Verification items for the finished model (mm, model axes). Face numbers are marked on the shaded views. A direction names the side the tool comes from. Round coordinates to 2 decimals unless told otherwise and drop trailing zeros. Write each loop counter-clockwise with the first axis right and the second up, starting at its lowest first coordinate (ties: lowest second). Pieces come first, ordered by that corner, then holes. Notation, with made-up numbers: (76.25, 62) -> (111.25, 62) arc R15 ccw to (111.25, 86) -> close; hole circle Ø6 at (-1.5, 88). An arc over 180 degrees is marked (long way). Answer as a JSON object with one key per item and string values. Group by question number.
(1) Gauge pin test, flat ends, axial feed: pin 1 Ø6 at (x, y) = (13.5, 41) entering from -Z; pin 2 Ø1.6 at (x, z) = (34.5, -47.5) entering from +Y; pin 3 Ø12 at (y, z) = (38.5, -49.5) entering from -X; pin 4 Ø10 at (x, z) = (22, -36) entering from -Y. Record the tip position at first contact, or that the pin passes through.
(2) Sectioned sample at B-B on z = -33.5. Record the cut outline in (x, y), and give its area (3 significant figures).
(3) Sectioned sample at C-C on x = 14.5. Record the cut outline in (y, z), and give its area (3 significant figures).
(4) Scan lines: L1, parallel to X at y = 42.75, z = -55.5; L2, parallel to Y at x = 14.5, z = -49; L3, parallel to X at y = 48.75, z = -42. Record each from-to range of solid material in increasing order. Write a range as from..to.
(5) Sectioned sample at A-A on x = 7. Record the cut outline in (y, z).
(6) Draft check along X on the marked faces 4, 5 and 6. Enter one of: released by +X, released by -X, zero draft, split by the parting line, or undercut.
(7) Set-up check for the marked faces 1, 2 and 3: record each of +Z, -Z, +X, -X, +Y, -Y from which the full face is reachable in a straight line by a thin tool's end or side.
(8) Sectioned sample at D-D on y = 51. Record the cut outline in (x, z), and give its area (3 significant figures).
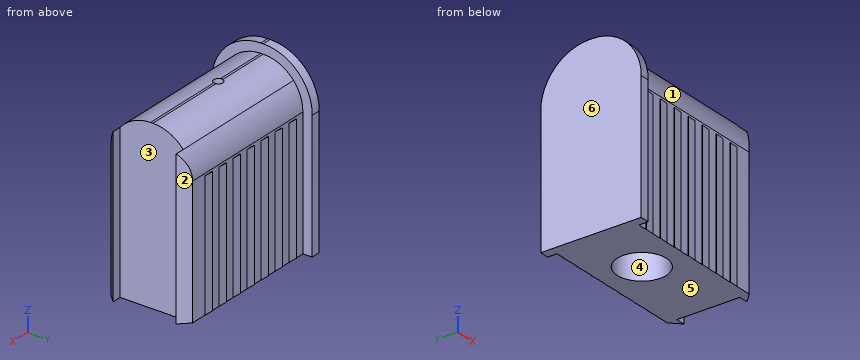
```python
from build123d import *

# Parameters (mm, degrees)
F1_DEPTH = 35.5
F2_DEPTH = 2
F3_DEPTH = 33.5
F4_R     = 5.25
F4_R_2   = 1
F5_DEPTH = 25
F6_DEPTH = 36
F7_DEPTH = 32.9782255751
F8_DEPTH = 27


with BuildPart() as f1:
    # F0 (on Right) → F1 (new body)
    with BuildSketch(Plane.YZ):
        with BuildLine():
            Line((49.4756655051, -63.7959514514), (51.4756655051, -63.7959514514))
            Line((51.4756655051, -63.7959514514), (51.4756655051, -36.2959514514))
            ThreePointArc((51.4756655051, -36.2959514514), (50.9600252165, -33.3804755039), (49.4756655051, -30.8187258763))
            Line((49.4756655051, -30.8187258763), (49.4756655051, -63.7959514514))
        make_face()
    extrude(amount=F1_DEPTH)



with BuildPart() as f1b:
    # F0 (on Right) → F1, piece 2 (new body)
    with BuildSketch(Plane.YZ):
        with BuildLine():
            Line((33.9756655051, -63.7959514514), (35.9756655051, -63.7959514514))
            Line((35.9756655051, -63.7959514514), (35.9756655051, -30.8187258763))
            ThreePointArc((35.9756655051, -30.8187258763), (34.4913057938, -33.3804755039), (33.9756655051, -36.2959514514))
            Line((33.9756655051, -36.2959514514), (33.9756655051, -63.7959514514))
        make_face()
    extrude(amount=F1_DEPTH)


with BuildPart() as f1_1:
    add(f1.part)

    add(f1b.part)  # F2 merges F1b
    # F0 (on Right) → F2 (join)
    with BuildSketch(Plane.YZ):
        with BuildLine():
            Line((51.4756655051, -36.2959514514), (51.4756655051, -63.7959514514))
            Line((51.4756655051, -63.7959514514), (53.4756655051, -63.7959514514))
            Line((53.4756655051, -63.7959514514), (53.4756655051, -36.2959514514))
            ThreePointArc((53.4756655051, -36.2959514514), (50.4002867076, -28.8713302489), (42.9756655051, -25.7959514514))
            Line((42.9756655051, -25.7959514514), (42.4756655051, -25.7959514514))
            ThreePointArc((42.4756655051, -25.7959514514), (35.0510443027, -28.8713302489), (31.9756655051, -36.2959514514))
            Line((31.9756655051, -36.2959514514), (31.9756655051, -63.7959514514))
            Line((31.9756655051, -63.7959514514), (33.9756655051, -63.7959514514))
            Line((33.9756655051, -63.7959514514), (33.9756655051, -36.2959514514))
            ThreePointArc((33.9756655051, -36.2959514514), (34.4913057938, -33.3804755039), (35.9756655051, -30.8187258763))
            ThreePointArc((35.9756655051, -30.8187258763), (38.8914234226, -28.5886037432), (42.4756655051, -27.7959514514))
            Line((42.4756655051, -27.7959514514), (42.9756655051, -27.7959514514))
            ThreePointArc((42.9756655051, -27.7959514514), (46.5599075877, -28.5886037432), (49.4756655051, -30.8187258763))
            ThreePointArc((49.4756655051, -30.8187258763), (50.9600252165, -33.3804755039), (51.4756655051, -36.2959514514))
        make_face()
        with BuildLine():
            Line((35.9756655051, -63.7959514514), (49.4756655051, -63.7959514514))
            Line((49.4756655051, -63.7959514514), (49.4756655051, -30.8187258763))
            ThreePointArc((49.4756655051, -30.8187258763), (46.5599075877, -28.5886037432), (42.9756655051, -27.7959514514))
            Line((42.9756655051, -27.7959514514), (42.4756655051, -27.7959514514))
            ThreePointArc((42.4756655051, -27.7959514514), (38.8914234226, -28.5886037432), (35.9756655051, -30.8187258763))
            Line((35.9756655051, -30.8187258763), (35.9756655051, -63.7959514514))
        make_face()
    extrude(amount=F2_DEPTH)

    # F0 (on Right) → F3 (join)
    with BuildSketch(Plane.YZ):
        with BuildLine():
            Line((35.9756655051, -63.7959514514), (49.4756655051, -63.7959514514))
            Line((49.4756655051, -63.7959514514), (49.4756655051, -30.8187258763))
            ThreePointArc((49.4756655051, -30.8187258763), (46.5599075877, -28.5886037432), (42.9756655051, -27.7959514514))
            Line((42.9756655051, -27.7959514514), (42.4756655051, -27.7959514514))
            ThreePointArc((42.4756655051, -27.7959514514), (38.8914234226, -28.5886037432), (35.9756655051, -30.8187258763))
            Line((35.9756655051, -30.8187258763), (35.9756655051, -63.7959514514))
        make_face()
    extrude(amount=F3_DEPTH)

    # F4 (on face) → F5 (cut)
    with BuildSketch(Plane(origin=(0, 0, -63.7959514514), x_dir=(1, 0, 0), z_dir=(0, 0, -1))):
        with Locations((14.5, -42.7256655051)):
            Circle(F4_R)
        with Locations((14.5, -42.7256655051)):
            Circle(F4_R_2, mode=Mode.SUBTRACT)
    extrude(amount=-F5_DEPTH, mode=Mode.SUBTRACT)

    # F6 (cut, through all): a face of the model
    f6_faces = [f1_1.faces().sort_by_distance(p)[0] for p in [
        (14.5, 42.7256655051, -63.7959514514),
    ]]
    extrude(f6_faces, amount=-F6_DEPTH, mode=Mode.SUBTRACT)

    # F4 (on face) → F7 (cut, through all)
    with BuildSketch(Plane(origin=(0, 0, -63.7959514514), x_dir=(1, 0, 0), z_dir=(0, 0, -1))):
        Polygon((35.5, -49.4756655051), (33.5, -51.4756655051), (35.5, -51.4756655051), align=None)
        Polygon((35.5, -33.9756655051), (33.5, -33.9756655051), (35.5, -35.9756655051), align=None)
    extrude(amount=-F7_DEPTH, mode=Mode.SUBTRACT)

    # F4 (on face) → F8 (join)
    with BuildSketch(Plane(origin=(0, 0, -63.7959514514), x_dir=(1, 0, 0), z_dir=(0, 0, -1))):
        Polygon((4, -51.5756655051), (6, -51.4756655051), (4, -51.4756655051), align=None)
        Polygon((8, -51.5756655051), (10, -51.4756655051), (8, -51.4756655051), align=None)
        Polygon((28, -51.5756655051), (30, -51.4756655051), (28, -51.4756655051), align=None)
        Polygon((24, -51.5756655051), (26, -51.4756655051), (24, -51.4756655051), align=None)
        Polygon((20, -51.5756655051), (22, -51.4756655051), (20, -51.4756655051), align=None)
        Polygon((16, -51.5756655051), (18, -51.4756655051), (16, -51.4756655051), align=None)
        Polygon((12, -51.5756655051), (14, -51.4756655051), (12, -51.4756655051), align=None)
        Polygon((28, -33.9756655051), (30, -33.9756655051), (28, -33.8756655051), align=None)
        Polygon((24, -33.9756655051), (26, -33.9756655051), (24, -33.8756655051), align=None)
        Polygon((20, -33.9756655051), (22, -33.9756655051), (20, -33.8756655051), align=None)
        Polygon((16, -33.9756655051), (18, -33.9756655051), (16, -33.8756655051), align=None)
        Polygon((12, -33.9756655051), (14, -33.9756655051), (12, -33.8756655051), align=None)
        Polygon((8, -33.9756655051), (10, -33.9756655051), (8, -33.8756655051), align=None)
        Polygon((4, -33.9756655051), (6, -33.9756655051), (4, -33.8756655051), align=None)
    extrude(amount=-F8_DEPTH)


solid = f1_1.part
```
Computed values:
{
 "1": {"pin 1": "z = -38.8", "pin 2": "y = 51.28", "pin 3": "x = 0", "pin 4": "y = 33.88"},
 "2": {"outline": "(0, 32.35) -> (2, 32.35) -> (2, 34.45) -> (33.97, 34.45) -> (35.5, 35.98) -> (33.5, 35.98) -> (33.5, 49.48) -> (35.5, 49.48) -> (33.97, 51) -> (2, 51) -> (2, 53.1) -> (0, 53.1) -> close; hole circle Ø2 at (14.5, 42.73)", "area": "564 mm2"},
 "3": {"outline": "(33.98, -63.8) -> (37.48, -63.8) -> (37.48, -38.8) -> (41.73, -38.8) -> (41.73, -27.83) arc R8.5 ccw to (33.98, -36.3) -> close; (43.73, -38.8) -> (47.98, -38.8) -> (47.98, -63.8) -> (51.48, -63.8) -> (51.48, -36.3) arc R8.5 ccw to (43.73, -27.83) -> close", "area": "315 mm2"},
 "4": {"L1": "0..9.25, 19.75..33.5", "L2": "33.98..37.48, 47.98..51.48", "L3": "0..33.5"},
 "5": {"outline": "(33.98, -63.8) -> (51.48, -63.8) -> (51.48, -36.3) arc R8.5 ccw to (42.98, -27.8) -> (42.48, -27.8) arc R8.5 ccw to (33.98, -36.3) -> close"},
 "6": {"face 4": "undercut", "face 5": "zero draft", "face 6": "released by -X"},
 "7": {"face 1": "+Z, +X, -Y", "face 2": "+Z, -Z, +X, +Y", "face 3": "+Z, -Z, +X"},
 "8": {"outline": "(0, -63.8) -> (33.98, -63.8) -> (33.98, -33.49) -> (2, -33.49) -> (2, -29.52) -> (0, -29.52) -> close", "area": "1,040 mm2"}
}
